Model file for the job. Use its own axes, mm. A direction names the side the tool comes from. Coordinates: 2 decimals unless noted, no trailing zeros. Write each loop counter-clockwise with the first axis right and the second up, starting at its lowest first coordinate (ties: lowest second). Pieces come first, ordered by that corner, then holes.
Q1. Pull direction Y, two halves, no side cores. Call faces 4 (the cylindrical face through (-15.12, -11.59, -0.79)), 5 (the flat face through (25, -19.045, 59)), 6 (the cylindrical face through (24.7, 21.33, 2.46)): released by +Y, released by -Y, zero draft, split by the parting line, or undercut.
Q2. Band-saw the part on D-D, the plane x = -13. Write the cut outline in (y, z).
Q3. Pin check, flat tips, straight feed: P1, Ø1.6, axis at x = -24.5, z = 71.5, coming from the -Y side (3 decimals); P2, Ø8, axis at x = -23.55, y = 23.55, coming from the -Z side; P3, Ø3, axis at x = 21, z = 32, coming from the -Y side. Stop position of each tip, or through.
Q4. Band-saw the part on A-A, the plane x = 0. Write the cut outline in (y, z), plus the area to 3 significant figures.
Q5. Which spindle directions (+Z, -Z, +X, -X, +Y, -Y) get a long thin tool onto all of the face, cutting with end or side? Do faces 1 (the flat face through (-24, 26.5, 5)), 2 (the flat face through (0, 4.5, -14)), 3 (the flat face through (4, -4, -1.6)). Say none if no direction does.
Q6. Drill centre lines: probe 1 along Y at (x, z) = (23.55, 2.55); probe 2 along Z at (x, y) = (-0.5, -17.5). Where is each one in solid material? Low to high.
Q7. Band-saw the part on B-B, the plane y = 0. Write the cut outline in (x, z).
Q8. Band-saw the part on C-C, the plane z = 56. Write the cut outline in (x, y), plus the area to 3 significant figures.
from build123d import *

# Parameters (mm, degrees)
SKETCH1_W           = 56.4
SKETCH1_H           = 56.4
SKETCH1_R           = 2.5
SKETCH1_R_2         = 19.05
SKETCH1_R_3         = 5
BOSS_EXTRUDE1_DEPTH = 112
SKETCH1_3_R         = 19.05
SKETCH1_3_R_2       = 5
BOSS_EXTRUDE2_DEPTH = 1.6
FILLET1_R           = 5
CUT_EXTRUDE1_DEPTH  = 107
FILLET2_R           = 1.5
SKETCH1_4_R         = 5
BOSS_EXTRUDE3_DEPTH = 24.2
SKETCH3_W           = 4.358898944
SKETCH3_H           = 0.854235542
CUT_EXTRUDE2_DEPTH  = 20


with BuildPart() as part:
    # Sketch1 → Boss-Extrude1 (new body)
    with BuildSketch(Plane.XY):
        Rectangle(SKETCH1_W, SKETCH1_H)
        with Locations((-23.55, -23.55)):
            Circle(SKETCH1_R, mode=Mode.SUBTRACT)
        with Locations((23.55, -23.55)):
            Circle(SKETCH1_R, mode=Mode.SUBTRACT)
        with Locations((23.55, 23.55)):
            Circle(SKETCH1_R, mode=Mode.SUBTRACT)
        with Locations((-23.55, 23.55)):
            Circle(SKETCH1_R, mode=Mode.SUBTRACT)
        Circle(SKETCH1_R_2, mode=Mode.SUBTRACT)
        Circle(SKETCH1_R_2)
        Circle(SKETCH1_R_3, mode=Mode.SUBTRACT)
        Circle(SKETCH1_R_3)
    extrude(amount=BOSS_EXTRUDE1_DEPTH)

    # Sketch1_3 → Boss-Extrude2 (add)
    with BuildSketch(Plane.XY):
        Circle(SKETCH1_3_R)
        Circle(SKETCH1_3_R_2, mode=Mode.SUBTRACT)
        Circle(SKETCH1_3_R_2)
    extrude(amount=-BOSS_EXTRUDE2_DEPTH)

    # Fillet1
    fillet1_edges = [part.edges().sort_by_distance(p)[0] for p in [
        (-28.2, -28.2, 56),
        (-28.2, 28.2, 56),
        (28.2, 28.2, 56),
        (28.2, -28.2, 56),
    ]]
    fillet(fillet1_edges, radius=FILLET1_R)

    # Sketch2 → Cut-Extrude1 (cut)
    with BuildSketch(Plane.XY.offset(112)):
        with BuildLine():
            Line((-23.55, 19.044974747), (-31.616752069, 19.044974747))
            Line((-31.616752069, 19.044974747), (-31.616752069, 32.365774456))
            Line((-31.616752069, 32.365774456), (-19.044974747, 32.365774456))
            Line((-19.044974747, 32.365774456), (-19.044974747, 23.55))
            ThreePointArc((-19.044974747, 23.55), (-20.364466094, 20.364466094), (-23.55, 19.044974747))
        make_face()
        with BuildLine():
            Line((19.044974747, 23.55), (19.044974747, 31.616752069))
            Line((19.044974747, 31.616752069), (32.365774456, 31.616752069))
            Line((32.365774456, 31.616752069), (32.365774456, 19.044974747))
            Line((32.365774456, 19.044974747), (23.55, 19.044974747))
            ThreePointArc((23.55, 19.044974747), (20.364466094, 20.364466094), (19.044974747, 23.55))
        make_face()
        with BuildLine():
            Line((23.55, -19.044974747), (31.616752069, -19.044974747))
            Line((31.616752069, -19.044974747), (31.616752069, -32.365774456))
            Line((31.616752069, -32.365774456), (19.044974747, -32.365774456))
            Line((19.044974747, -32.365774456), (19.044974747, -23.55))
            ThreePointArc((19.044974747, -23.55), (20.364466094, -20.364466094), (23.55, -19.044974747))
        make_face()
        with BuildLine():
            Line((-19.044974747, -23.55), (-19.044974747, -31.616752069))
            Line((-19.044974747, -31.616752069), (-32.365774456, -31.616752069))
            Line((-32.365774456, -31.616752069), (-32.365774456, -19.044974747))
            Line((-32.365774456, -19.044974747), (-23.55, -19.044974747))
            ThreePointArc((-23.55, -19.044974747), (-20.364466094, -20.364466094), (-19.044974747, -23.55))
        make_face()
    extrude(amount=-CUT_EXTRUDE1_DEPTH, mode=Mode.SUBTRACT)

    # Fillet2
    fillet2_edges = [part.edges().sort_by_distance(p)[0] for p in [
        (28.2, -19.044974747, 58.5),
        (19.044974747, -28.2, 58.5),
        (-19.044974747, -28.2, 58.5),
        (-28.2, -19.044974747, 58.5),
        (-28.2, 19.044974747, 58.5),
        (-19.044974747, 28.2, 58.5),
        (19.044974747, 28.2, 58.5),
        (28.2, 19.044974747, 58.5),
    ]]
    fillet(fillet2_edges, radius=FILLET2_R)

    # Sketch1_4 → Boss-Extrude3 (add)
    with BuildSketch(Plane.XY):
        Circle(SKETCH1_4_R)
    extrude(amount=-BOSS_EXTRUDE3_DEPTH)

    # Sketch3 → Cut-Extrude2 (cut)
    with BuildSketch(Plane(origin=(0, 0, -24.2), x_dir=(-1, 0, 0), z_dir=(0, 0, -1))):
        with Locations((0, 4.927117771)):
            Rectangle(SKETCH3_W, SKETCH3_H)
    extrude(amount=-CUT_EXTRUDE2_DEPTH, mode=Mode.SUBTRACT)


solid = part.part
Answer sheet:
1. face 4: split by the parting line
1. face 5: released by -Y
1. face 6: undercut
2. outline: (-28.2, 0) - (-13.92, 0) - (-13.92, -1.6) - (13.92, -1.6) - (13.92, 0) - (28.2, 0) - (28.2, 112) - (-28.2, 112) - close
3. P1: stops at y = -19.045
3. P2: stops at z = 0
3. P3: stops at y = -21.58
4. outline: (-28.2, 0) - (-19.05, 0) - (-19.05, -1.6) - (-5, -1.6) - (-5, -24.2) - (4.5, -24.2) - (4.5, -4.2) - (5, -4.2) - (5, -1.6) - (19.05, -1.6) - (19.05, 0) - (28.2, 0) - (28.2, 112) - (-28.2, 112) - close
4. area: 6,590 mm2
5. face 1: +Z, -X, +Y
5. face 2: -Z, +X, -X, +Y
5. face 3: -Z
6. probe 1: y = -28.19 to -26.05, -21.05 to 21.05, 26.05 to 28.19
6. probe 2: z = -1.6 to 112
7. outline: (-28.2, 0) - (-19.05, 0) - (-19.05, -1.6) - (-5, -1.6) - (-5, -24.2) - (5, -24.2) - (5, -1.6) - (19.05, -1.6) - (19.05, 0) - (28.2, 0) - (28.2, 112) - (-28.2, 112) - close
8. outline: (-28.2, -17.54) arc R1.5 ccw to (-26.7, -19.04) - (-23.55, -19.04) arc R4.51 cw to (-19.04, -23.55) - (-19.04, -26.7) arc R1.5 ccw to (-17.54, -28.2) - (17.54, -28.2) arc R1.5 ccw to (19.04, -26.7) - (19.04, -23.55) arc R4.51 cw to (23.55, -19.04) - (26.7, -19.04) arc R1.5 ccw to (28.2, -17.54) - (28.2, 17.54) arc R1.5 ccw to (26.7, 19.04) - (23.55, 19.04) arc R4.51 cw to (19.04, 23.55) - (19.04, 26.7) arc R1.5 ccw to (17.54, 28.2) - (-17.54, 28.2) arc R1.5 ccw to (-19.04, 26.7) - (-19.04, 23.55) arc R4.51 cw to (-23.55, 19.04) - (-26.7, 19.04) arc R1.5 ccw to (-28.2, 17.54) - close
8. area: 2,860 mm2
